Autodesk Inventor part; units mm, degrees
ref_plane "YZ Plane" through (0, 0, 0) normal (1, 0, 0) x (0, 1, 0)
ref_plane "XZ Plane" through (0, 0, 0) normal (0, 1, 0) x (-1, 0, 0)
ref_plane "XY Plane" through (0, 0, 0) normal (0, 0, 1) x (1, 0, 0)
sketch "JoystickMount" plane through (0, 0, 0) normal (0, 0, 1) x (1, 0, 0)
  line L0 (-49, 26.5) -> (49, 26.5)
  line L1 (49, 26.5) -> (49, -26.5)
  line L2 (49, -26.5) -> (-49, -26.5)
  line L3 (-49, -26.5) -> (-49, 26.5)
  point P0 (0, 0)
  point P1 (-49, 0)
  point P2 (0, 26.5)
  point P3 (0, -26.5)
  point P4 (49, 0)
  dimension "d0" = 53
  dimension "d2" = 98
extrude "JoystickMountPlate" add sketch "JoystickMount" against normal blind 2
fillet "MountPlateCornerFillet" radius 2 4 edges at (49, 26.5, -1) (-49, 26.5, -1) (-49, -26.5, -1) (49, -26.5, -1)
sketch "BodySketch" plane through (0, 0, -2) normal (0, 0, -1) x (-1, 0, 0)
  line L0 (-32.5, 31) -> (32.5, 31)
  line L1 (32.5, 31) -> (32.5, -31)
  line L2 (32.5, -31) -> (-32.5, -31)
  line L3 (-32.5, -31) -> (-32.5, 31)
  point P0 (0, 0)
  point P1 (-32.5, 0)
  point P2 (0, 31)
  dimension "d6" = 65
  dimension "d8" = 62
extrude "JoystickBody" add sketch "BodySketch" along normal blind 36
sketch "JoystickPostCenter" plane through (0, 0, 0) normal (0, 0, 1) x (1, 0, 0)
  circle A0 centre (0, 0) radius 4
  dimension "d11" = 8
extrude "Shaft" add sketch "JoystickPostCenter" along normal blind 32
sketch "ThreadSketch" plane through (0, 0, 32) normal (0, 0, 1) x (1, 0, 0)
  circle A0 centre (0, 0) radius 4
  circle A1 centre (0, 0) radius 2.5
  dimension "d14" = 5
extrude "ShaftScrew" add sketch "ThreadSketch" along normal blind 10 contours A1
thread "ShaftThread"
sketch "MountHoles" plane through (0, 0, 0) normal (0, 0, 1) x (1, 0, 0)
  circle A0 centre (0, 0) radius 4
  line L0 (47, -26.5) -> (-47, -26.5)
  line L1 (-42.5, 20.25) -> (-42.5, -20.25) construction
  line L2 (-42.5, -20.25) -> (42.5, -20.25) construction
  point P0 (42.5, 20.25)
  point P1 (-42.5, 0)
  point P2 (0, -20.25)
  dimension "d44" = 40.5
  dimension "d46" = 85
hole "MountingHoles" at (-42.5, 20.25, 0) at (-42.5, -20.25, 0) at (42.5, -20.25, 0) at (42.5, 20.25, 0) direction (0, 0, -1) diameter 4.5 end through all
properties part number "JLF-TP-8YT_body" material "Steel AISI 4620"
Geometry: final body of the model. Coordinates: model frame, mm. A direction names the side the tool comes from. Round coordinates to 2 decimals unless told otherwise and drop trailing zeros. Order: outer loops, then holes, each group sorted by start corner. A loop starts at its lowest first (then second) coordinate and runs counter-clockwise, first axis right, second up. Notation, with made-up numbers: (-33, 30) -> (-15, 30) arc R20 ccw to (-15, 37) -> close; hole circle Ø8 at (64, -3.75). An arc over 180 degrees is marked (long way). Put each result on its own line as item: value. Start each with the question number.
Q1. Reachability of faces 1 (the flat face through (2, 2, 32)), 2 (the flat face through (0, -29, -2)), 3 (the flat face through (-41, 0, -2)), 4 (the flat face through (32.5, 0, -20)) from +Z, -Z, +X, -X, +Y, -Y: full face, straight path, thin tool, end or side. Return the list, or none.
Q2. Line query: probe 1 along X at (y, z) = (20.25, -1.4); probe 2 along Y at (x, z) = (-42.5, -1); probe 3 along Z at (x, y) = (18, -25.5). Output: solid intervals per line, ascending.
Q3. Section D-D on x = 15. Return the cut outline in (y, z), and give its area (3 significant figures).
Q4. First-contact query: pin 1 (12 mm diameter, centred on y = 2, z = -7, fed in from +X); pin 2 (6 mm diameter, centred on x = -2, z = 26, fed in from -Y); pin 3 (1 mm diameter, centred on y = 0, z = 13.5, fed in from -X); pin 4 (2 mm diameter, centred on x = -12.5, y = 29.5, fed in from +Z). Flat tips, straight axial feed; report the tip coordinate or a pass-through.
Q5. Section B-B on x = 0. Return the cut outline in (y, z), and give its area (3 significant figures).
Q6. Section A-A on y = 20.25. Return the cut outline in (x, z), and give its area (3 significant figures).
Q7. Section C-C on y = -14.5. Return the cut outline in (x, z), and give its area (3 significant figures).
Q8. Pull-direction query (Y, two-part tool) for faces 5 (the cylindrical face through (-44.397, 19.04, -1.014)), 6 (the flat face through (0, 0, -38)), 7 (the flat face through (0, -31, -20)); classes: +Y half, -Y half, draft (parallel to the pull), parting line (faces both ways), or undercut.
Ans:
1. face 1: +Z
1. face 2: +Z, +X, -X, -Y
1. face 3: -Z, -X, +Y, -Y
1. face 4: -Z, +X, +Y, -Y
2. probe 1: x = -49 to -44.75, -40.25 to 40.25, 44.75 to 49
2. probe 2: y = -26.5 to -22.5, -18 to 18, 22.5 to 26.5
2. probe 3: z = -38 to 0
3. outline: (-31, -38) -> (31, -38) -> (31, -2) -> (26.5, -2) -> (26.5, 0) -> (-26.5, 0) -> (-26.5, -2) -> (-31, -2) -> close
3. area: 2,340 mm2
4. pin 1: stops at x = 49
4. pin 2: stops at y = -4
4. pin 3: stops at x = -4
4. pin 4: stops at z = -2
5. outline: (-31, -38) -> (31, -38) -> (31, -2) -> (26.5, -2) -> (26.5, 0) -> (4, 0) -> (4, 32) -> (2.5, 32) -> (2.5, 42) -> (-2.5, 42) -> (-2.5, 32) -> (-4, 32) -> (-4, 0) -> (-26.5, 0) -> (-26.5, -2) -> (-31, -2) -> close
5. area: 2,640 mm2
6. outline: (-49, -2) -> (-44.75, -2) -> (-44.75, 0) -> (-49, 0) -> close; (-40.25, -2) -> (-32.5, -2) -> (-32.5, -38) -> (32.5, -38) -> (32.5, -2) -> (40.25, -2) -> (40.25, 0) -> (-40.25, 0) -> close; (44.75, -2) -> (49, -2) -> (49, 0) -> (44.75, 0) -> close
6. area: 2,520 mm2
7. outline: (-49, -2) -> (-32.5, -2) -> (-32.5, -38) -> (32.5, -38) -> (32.5, -2) -> (49, -2) -> (49, 0) -> (-49, 0) -> close
7. area: 2,540 mm2
8. face 5: undercut
8. face 6: draft
8. face 7: -Y half
